```python
from build123d import *

# Parameters (mm, degrees)
SKETCH_2_R          = 11.601145783
CUT_EXTRUDE_1_DEPTH = 10


with BuildPart() as part:
    # Эскиз1 → Повернуть1 (revolve)
    with BuildSketch(Plane.XY):
        with BuildLine():
            Line((-8, -6.973192061), (-6, -6.973192061))
            Line((-6, -6.973192061), (-6, -0.973192061))
            add(Edge.make_bspline(
                [(-6, -0.973192061), (-5.270413842, 0.380623503), (-3.5, 0.326807939)],
                knots=[0, 0, 0, 1, 1, 1], degree=2))
            Line((-3.5, 0.326807939), (-3.5, 0.526807939))
            Line((-3.5, 0.526807939), (-4.5, 0.526807939))
            ThreePointArc((-4.5, 0.526807939), (-5.914213562, -0.058978499), (-6.5, -1.473192061))
            Line((-6.5, -1.473192061), (-6.5, -3.473192061))
            Line((-6.5, -3.473192061), (-8, -3.473192061))
            Line((-8, -3.473192061), (-8, -6.973192061))
        make_face()
    revolve(axis=Axis((0, -7.792035126, 0), (0, 1, 0)))

    # Эскиз2 → Вырез-Вытянуть1 (cut)
    with BuildSketch(Plane(origin=(0, -3.473192061, 0), x_dir=(1, 0, 0), z_dir=(0, 1, 0))):
        Circle(SKETCH_2_R)
        Polygon((0, 8), (6.92820323, 4), (6.92820323, -4), (0, -8), (-6.92820323, -4), (-6.92820323, 4), align=None, mode=Mode.SUBTRACT)
    extrude(amount=-CUT_EXTRUDE_1_DEPTH, mode=Mode.SUBTRACT)


solid = part.part
```
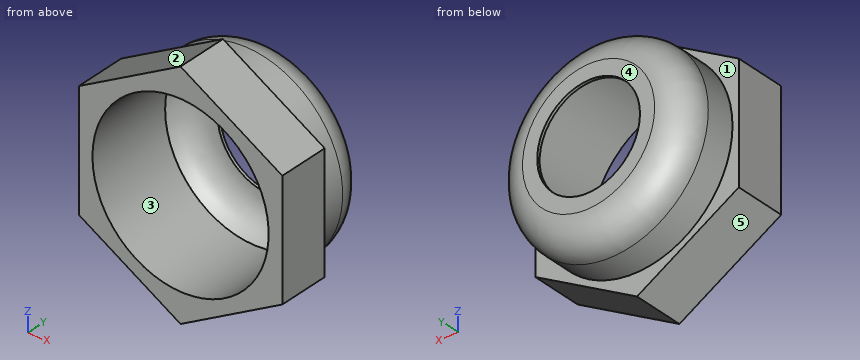
For this review, take the finished solid that the model builds, in its own axes (mm). Face numbers are marked on the shaded views. A direction names the side the tool comes from. Round coordinates to 2 decimals unless told otherwise and drop trailing zeros. Write each loop counter-clockwise with the first axis right and the second up, starting at its lowest first coordinate (ties: lowest second). Pieces come first, ordered by that corner, then holes. Notation, with made-up numbers: M 42.25,-39 L 46.25,-39 A13 cw 46.25,-33 Z; hole C 22,-25.75 d6. An arc over 180 degrees is marked long. One line per item, written item: value. Start each with the question number.
(1) The part is to be moulded in two halves that separate along X. For the marked faces 3, 4 and 5, say which applies: released by +X, released by -X, zero draft, split by the parting line, or undercut.
(2) Machinability: for the marked faces 1 and 2, which of the approach directions +Z, -Z, +X, -X, +Y, -Y give a long, thin tool a straight path to every point of the face, cutting with its end or side? Answer none if there is none.
(3) Wall thickness on line 1 (Z direction, x = -1, y = -4.5); line 2 (Z direction, x = -5.5, y = -5.25); line 3 (X direction, y = -1.75, z = -0.25): over which ranges is each line inside the solid? List them lowest first.
(4) Insertion check: pin 1 (3 mm diameter, centred on y = -4, z = -6, fed in from +X); pin 2 (1 mm diameter, centred on x = 1, y = -0.5, fed in from +Z); pin 3 (1.5 mm diameter, centred on x = 0.5, y = -6, fed in from -Z). Each pin has a flat end and moves straight along its axis. Give the tip position at first contact, or say it passes through.
(5) We need section C-C (y = -1.25). Give the boundary of the cut face in (x, z), and give its area (3 significant figures).
(6) We need section A-A (y = -4.5). Give the boundary of the cut face in (x, z), and give its area (3 significant figures).
(7) We need section B-B (y = -2.5). Give the boundary of the cut face in (x, z), and give its area (3 significant figures).
Result:
1. face 3: undercut
1. face 4: zero draft
1. face 5: released by -X
2. face 1: +Y
2. face 2: +Z, -X, +Y, -Y
3. line 1: -7.42 to -5.92, 5.92 to 7.42
3. line 2: -4.82 to -2.4, 2.4 to 4.82
3. line 3: -6.5 to -5.99, 5.99 to 6.5
4. pin 1: x = 6.06
4. pin 2: z = 6.38
4. pin 3: z = -8
5. outline: C 0,0 d12.98; hole C 0,0 d12
5. area: 19.1 mm²
6. outline: M -6.93,-4 L 0,-8 L 6.93,-4 L 6.93,4 L 0,8 L -6.93,4 Z; hole C 0,0 d12
6. area: 53.2 mm²
7. outline: C 0,0 d13; hole C 0,0 d12
7. area: 19.6 mm²
